```python
from build123d import *

# Parameters (mm, degrees)
BOSS_EXTRUDE1_DEPTH      = 25.4
BOSS_EXTRUDE1_DEPTH_BACK = 8.255
SKETCH1_W                = 44.45
SKETCH1_H                = 31.75
CUT_EXTRUDE1_DEPTH       = 7.9375
SKETCH3_R                = 3.175
CUT_EXTRUDE2_DEPTH       = 65.160143586
SKETCH4_R                = 1.89865
CUT_EXTRUDE4_DEPTH       = 4.7625
FILLET1_R                = 2.54
CUT_EXTRUDE5_DEPTH       = 10.4775
FILLET2_R                = 7.62


with BuildPart() as part:
    # Sketch1 → Boss-Extrude1 (new, two sides: drawn at the far end of the back side and taken through both)
    with BuildSketch(Plane(origin=(0, 0, 0), x_dir=(0, 0, -1), z_dir=(1, 0, 0)).offset(-BOSS_EXTRUDE1_DEPTH_BACK)):
        with Locations((22.225, -15.875)):
            Rectangle(SKETCH1_W, SKETCH1_H)
    extrude(amount=BOSS_EXTRUDE1_DEPTH + BOSS_EXTRUDE1_DEPTH_BACK)

    # Sketch2 → Cut-Extrude1 (cut)
    with BuildSketch(Plane.ZY.offset(8.255)):
        Polygon((-18.558825791, -15.875), (-14.892651581, -9.525), (-18.558825791, -3.175), (-25.891174209, -3.175), (-29.557348419, -9.525), (-25.891174209, -15.875), align=None)
    extrude(amount=-CUT_EXTRUDE1_DEPTH, mode=Mode.SUBTRACT)

    # Sketch3 → Cut-Extrude2 (cut, through all)
    with BuildSketch(Plane(origin=(25.4, 0, 0), x_dir=(0, 0, -1), z_dir=(1, 0, 0))):
        with Locations((22.225, -9.525)):
            Circle(SKETCH3_R)
    extrude(amount=-CUT_EXTRUDE2_DEPTH, mode=Mode.SUBTRACT)

    # Sketch4 → Cut-Extrude4 (cut)
    with BuildSketch(Plane.XY):
        with Locations((9.525, -15.875)):
            Circle(SKETCH4_R)
    cut_extrude4 = extrude(amount=-CUT_EXTRUDE4_DEPTH, mode=Mode.SUBTRACT)

    # Mirror3: Cut-Extrude4 across plane
    add(cut_extrude4.mirror(Plane.XY.offset(-22.225)), mode=Mode.SUBTRACT)

    # Fillet1
    fillet1_edges = [part.edges().sort_by_distance(p)[0] for p in [
        (8.5725, 0, 0),
        (8.5725, 0, -44.45),
        (8.5725, -31.75, -44.45),
        (8.5725, -31.75, 0),
    ]]
    fillet(fillet1_edges, radius=FILLET1_R)

    # Sketch5 → Cut-Extrude5 (cut)
    with BuildSketch(Plane.ZY.offset(8.255)):
        with BuildLine():
            Line((-44.45, -2.54), (-44.45, -29.21))
            ThreePointArc((-44.45, -29.21), (-43.706051224, -31.006051224), (-41.91, -31.75))
            Line((-41.91, -31.75), (-2.54, -31.75))
            ThreePointArc((-2.54, -31.75), (-0.743948776, -31.006051224), (0, -29.21))
            Line((0, -29.21), (0, -2.54))
            ThreePointArc((0, -2.54), (-0.743948776, -0.743948776), (-2.54, 0))
            Line((-2.54, 0), (-16.725738686, 0))
            Line((-16.725738686, 0), (-11.226477372, -9.525))
            Line((-11.226477372, -9.525), (-16.725738686, -19.05))
            Line((-16.725738686, -19.05), (-27.724261314, -19.05))
            Line((-27.724261314, -19.05), (-33.223522628, -9.525))
            Line((-33.223522628, -9.525), (-27.724261314, 0))
            Line((-27.724261314, 0), (-41.91, 0))
            ThreePointArc((-41.91, 0), (-43.706051224, -0.743948776), (-44.45, -2.54))
        make_face()
    extrude(amount=-CUT_EXTRUDE5_DEPTH, mode=Mode.SUBTRACT)

    # Fillet2
    fillet2_edges = [part.edges().sort_by_distance(p)[0] for p in [
        (2.2225, -4.7625, -30.473891971),
        (2.2225, -14.2875, -30.473891971),
        (2.2225, -19.05, -22.225),
        (2.2225, -14.2875, -13.976108029),
        (2.2225, -4.7625, -13.976108029),
    ]]
    fillet(fillet2_edges, radius=FILLET2_R)


solid = part.part
```
Verification items for the finished model (mm, model axes). A direction names the side the tool comes from. Coordinates: 2 decimals unless noted, no trailing zeros. Write each loop counter-clockwise with the first axis right and the second up, starting at its lowest first coordinate (ties: lowest second). Pieces come first, ordered by that corner, then holes. Notation, with made-up numbers: M -21.5,-27.75 L 30.5,-27.75 A24 ccw 30.5,-17.75 Z; hole C 71.5,25 d5. An arc over 180 degrees is marked long. Answer as a JSON object with one key per item and string values. Group by question number.
(1) Tool access check on faces 1 (the face through (-4, -3.175, -22)), 2 (the face through (0.892, -22.368, -22.364)), 3 (the face through (-8.255, -3, -22)), 4 (the face through (-6.85, -4.7, -14.01)), 5 (the face through (-6.846, -4.829, -30.512)). Record the directions out of +Z, -Z, +X, -X, +Y, -Y that give a thin tool (end or side, any length) a straight path to the whole face; none if there is none.
(2) Cross-section at C-C, the plane y = -27.5. Record the cut outline in (x, z).
(3) Release check for a two-part mould opening along Y. For faces 6 (the face through (9, -16, -39.688)), 7 (the face through (7.63, -15.79, -2.35)), 8 (the face through (14, -31.75, -22)), 9 (the face through (13.973, -0.724, -43.686)) record: +Y half, -Y half, draft (parallel to the pull), parting line (faces both ways), or undercut.
(4) Gauge pin test, flat ends, axial feed: pin 1 (1.4 mm diameter, centred on x = -7, z = -20, fed in from -Y); pin 2 (5 mm diameter, centred on x = 9.525, y = -15.875, fed in from -Z); pin 3 (2 mm diameter, centred on x = -4.5, y = -9, fed in from +Z); pin 4 (1 mm diameter, centred on y = -6.5, z = -24, fed in from -X). Record the tip position at first contact, or that the pin passes through.
(5) Cross-section at A-A, the plane x = 16. Record the cut outline in (y, z) (3 decimals).
(6) Material ranges on line 1 (X direction, y = -3.5, z = -39.5); line 2 (Y direction, x = 10, z = -21); line 3 (Z direction, x = 12.5, y = -7), recorded low to high.
(7) Cross-section at D-D, the plane x = 1.5. Record the cut outline in (y, z) (3 decimals), and give its area (3 significant figures).
Reply:
{
 "1": {"face 1": "-X", "face 2": "+Z, -Z, -X, -Y", "face 3": "+Z, -Z, -X, +Y, -Y", "face 4": "+Z, -X, +Y", "face 5": "-Z, -X, +Y"},
 "2": {"outline": "M 2.22,-44.45 L 25.4,-44.45 L 25.4,0 L 2.22,0 Z"},
 "3": {"face 6": "undercut", "face 7": "undercut", "face 8": "-Y half", "face 9": "+Y half"},
 "4": {"pin 1": "y = -19.05", "pin 2": "z = -44.45", "pin 3": "z = -10.99", "pin 4": "x = -0.32"},
 "5": {"outline": "M -31.75,-41.91 A2.54 ccw -29.21,-44.45 L -2.54,-44.45 A2.54 ccw 0,-41.91 L 0,-2.54 A2.54 ccw -2.54,0 L -29.21,0 A2.54 ccw -31.75,-2.54 Z; hole C -9.525,-22.225 d6.35"},
 "6": {"line 1": "2.22 to 25.4", "line 2": "-31.75 to -12.45, -6.6 to 0", "line 3": "-44.45 to -24.15, -20.3 to 0"},
 "7": {"outline": "M -23.431,-30.254 L -9.525,-38.283 L 0,-32.783 L 0,-11.667 L -9.525,-6.167 L -23.431,-14.196 Z; hole C -9.525,-22.225 d6.35", "area": "557 mm²"}
}
